The listing builds one solid part. Answer for the finished solid, in the listing's coordinates (mm). Face numbers are marked on the shaded views. A direction names the side the tool comes from. Round coordinates to 2 decimals unless told otherwise and drop trailing zeros. Write each loop counter-clockwise with the first axis right and the second up, starting at its lowest first coordinate (ties: lowest second). Pieces come first, ordered by that corner, then holes. Notation, with made-up numbers: (0, 60.5) - (44, 60.5) arc R28 ccw to (44, 78.5) - close; hole circle Ø1 at (41.5, 80.5). An arc over 180 degrees is marked (long way). Return JSON: item names as keys, results as strings. Group by question number.
(1) Find the intervals of material crossed by line 1 along X through (y, z) = (17.5, 6); line 2 along Y through (x, z) = (-15, 9); line 3 along Y through (x, z) = (-8, 11), in increasing order. Write a range as [from, to].
(2) Determine the mould class of the marked faces 3, 4 and 5 for opening direction Y: +Y half, -Y half, draft (parallel to the pull), parting line (faces both ways), or undercut.
(3) Which of the six approach directions +Z, -Z, +X, -X, +Y, -Y give full straight-line access (tool end or side, diameter ignored) to the marked faces 1 and 2?
(4) Section D-D, the plane y = 5.5 is taken. Write down the section's boundary in (x, z).
(5) Each of these flat-tipped pins is pushed along its axis until it touches: pin 1 (4 mm diameter, centred on x = -10, z = 7.5, fed in from +Y); pin 2 (3 mm diameter, centred on x = 18, z = 2, fed in from +Y); pin 3 (3 mm diameter, centred on x = -10, y = 27.5, fed in from +Z); pin 4 (1 mm diameter, centred on y = 11.5, z = 7.5, fed in from -X). Where does it stop, or does it pass through?
(6) Section C-C, the plane z = 8.5 is taken. Write down the section's boundary in (x, y), then the cut area to 3 significant figures.
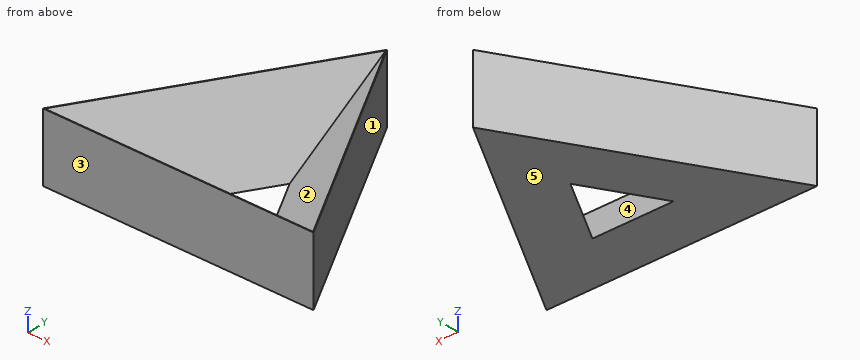
```python
from build123d import *

# Parameters (mm, degrees)
F1_DEPTH = 12.7
F2_SIZE2 = 10.15999
F2_SIZE  = 12.69999


# Not quite as in the source:
# - a fillet or chamfer is up to 0.001 mm smaller than in the source, because OpenCascade refuses the exact size


with BuildPart() as f1:
    # F0 (on Top) → F1 (new body)
    with BuildSketch(Plane.XY):
        Polygon((0, 43.9940905122), (-25.4, 0), (-7.62, 10.2652877862), (0, 23.4635149399), align=None)
        Polygon((7.62, 10.2652877862), (25.4, 0), (0, 43.9940905122), (0, 23.4635149399), align=None)
        Polygon((-7.62, 10.2652877862), (-25.4, 0), (25.4, 0), (7.62, 10.2652877862), align=None)
    extrude(amount=F1_DEPTH)

    # F2 (size 12.7 and 10.16 in the source; OpenCascade refuses exactly that, so slightly less here)
    f2_edges = [f1.edges().sort_by_distance(p)[0] for p in [
        (0, 10.265288, 12.7),
        (-3.81, 16.864401, 12.7),
        (3.81, 16.864401, 12.7),
    ]]
    chamfer(f2_edges, length=F2_SIZE, length2=F2_SIZE2)


solid = f1.part
```
Working result:
{
 "1": {"line 1": "x = [-15.3, -8.99], [8.99, 15.3]", "line 2": "y = [0, 3.07], [11.88, 18.01]", "line 3": "y = [0, 1.47], [27.21, 30.14]"},
 "2": {"face 3": "-Y half", "face 4": "undercut", "face 5": "draft"},
 "3": {"face 1": "+Z, -Z, +X, +Y", "face 2": "+Z"},
 "4": {"outline": "(-22.22, 0) - (22.22, 0) - (22.22, 12.7) - (22.1, 12.7) - (15.87, 5.96) - (-15.87, 5.96) - (-22.1, 12.7) - (-22.22, 12.7) - close"},
 "5": {"pin 1": "stops at y = 30.14", "pin 2": "stops at y = 15.42", "pin 3": "stops at z = 12.7", "pin 4": "stops at x = -19.05"},
 "6": {"outline": "(-25.4, 0) - (25.4, 0) - (0, 43.99) - close; hole (-19.4, 3.47) - (19.4, 3.47) - (0, 37.06) - close", "area": "466 mm^2"}
}
